Work out the finished part from the listing and answer in its coordinate system (mm). A direction names the side the tool comes from. Give positions to 0.01 mm unless a question says otherwise; leave off trailing zeros. Loops run counter-clockwise (first coordinate to the right, second up) from the corner with the lowest first, then second, coordinate; pieces in that order, holes last. Notation, with made-up numbers: (56.5, 52.25) - (67.5, 52.25) arc R28 cw to (67.5, 78.25) - close; hole circle Ø6 at (89.5, -36.5). An arc over 180 degrees is marked (long way). One line per item, written item: value.
from build123d import *

# Parameters (mm, degrees)
BOSS_EXTRUDE1_DEPTH = 254
SKETCH1_3_W         = 762
SKETCH1_3_H         = 254
BOSS_EXTRUDE2_DEPTH = 508
SKETCH1_4_W         = 1270
SKETCH1_4_H         = 254
BOSS_EXTRUDE3_DEPTH = 1016
SKETCH2_W           = 254
SKETCH2_H           = 254
CUT_EXTRUDE1_DEPTH  = 254


with BuildPart() as part:
    # Sketch1 → Boss-Extrude1 (new body)
    with BuildSketch(Plane(origin=(0, 0, 0), x_dir=(1, 0, 0), z_dir=(0, 1, 0))):
        Polygon((0, 1016), (0, 254), (762, 254), (762, 0), (1016, 0), (1524, 508), (1524, 762), (254, 762), (254, 1016), align=None)
    extrude(amount=BOSS_EXTRUDE1_DEPTH)

    # Sketch1<3> → Boss-Extrude2 (add)
    with BuildSketch(Plane(origin=(0, 0, 0), x_dir=(1, 0, 0), z_dir=(0, 1, 0))):
        with Locations((381, 127)):
            Rectangle(SKETCH1_3_W, SKETCH1_3_H)
    extrude(amount=BOSS_EXTRUDE2_DEPTH)

    # Sketch1<4> → Boss-Extrude3 (add)
    with BuildSketch(Plane(origin=(0, 0, 0), x_dir=(1, 0, 0), z_dir=(0, 1, 0))):
        with Locations((889, 889)):
            Rectangle(SKETCH1_4_W, SKETCH1_4_H)
    extrude(amount=BOSS_EXTRUDE3_DEPTH)

    # Sketch2 → Cut-Extrude1 (cut)
    with BuildSketch(Plane.XY.offset(-762)):
        Polygon((254, 254), (762, 1016), (254, 1016), align=None)
        with Locations((1143, 635)):
            Rectangle(SKETCH2_W, SKETCH2_H)
    extrude(amount=-CUT_EXTRUDE1_DEPTH, mode=Mode.SUBTRACT)


solid = part.part
1. The mould has two halves that part along Z. Classify faces 4 (the flat face through (762, 379, -125)), 5 (the flat face through (501, 250, 0)), 6 (the flat face through (751, 254, -515)), 7 (the flat face through (921, 388, -1016)): released by +Z, released by -Z, zero draft, split by the parting line, or undercut.
Output:
face 4: zero draft
face 5: released by +Z
face 6: undercut
face 7: released by -Z
2. For faces 1 (the flat face through (1141, 762, -887)), 2 (the flat face through (376, 379, -254)), 3 (the flat face through (504.444, 629.666, -887.222)), determine the directions among +Z, -Z, +X, -X, +Y, -Y from which every point of the face is accessible in a straight line to the end or side of a thin tool.
Output:
face 1: +Z, -Z
face 2: +X, -X, +Y
face 3: -Z, -X, +Y
3. Find the intervals of material crossed by line 1 along Y through (x, z) = (516, -386); line 2 along Z through (x, y) = (1195, 305); line 3 along X through (y, z) = (438, -164), in increasing order.
Output:
line 1: y = 0 to 254
line 2: z = -1016 to -762
line 3: x = 0 to 762
4. Section B-B (y = 398) is taken. Write down the section's boundary in (x, z), and give its area (3 significant figures).
Output:
outline: (0, -254) - (762, -254) - (762, 0) - (0, 0) - close; (350, -1016) - (1524, -1016) - (1524, -762) - (350, -762) - close
area: 492,000 mm²
5. Flat-ended cylindrical pins translate along their axes: pin 1 Ø10 at (y, z) = (167, -105) entering from +X; pin 2 Ø3 at (x, z) = (168, -579) entering from +Y. Find the tip coordinate at first contact, or state that the pin passes through.
Output:
pin 1: stops at x = 1126
pin 2: stops at y = 254
6. Section C-C (z = -224.5) is taken. Write down the section's boundary in (x, y).
Output:
outline: (0, 0) - (1240.5, 0) - (1240.5, 254) - (762, 254) - (762, 508) - (0, 508) - close
7. Section D-D (x = 418.5) is taken. Write down the section's boundary in (y, z).
Output:
outline: (0, -1016) - (500.75, -1016) - (500.75, -762) - (254, -762) - (254, -254) - (508, -254) - (508, 0) - (0, 0) - close
8. Section A-A (x = 1169) is taken. Write down the section's boundary in (y, z).
Output:
outline: (0, -1016) - (508, -1016) - (508, -762) - (254, -762) - (254, -153) - (0, -153) - close; (762, -1016) - (1016, -1016) - (1016, -762) - (762, -762) - close
